Can you work these out from the model? Positions are in its coordinate system, mm. A direction names the side the tool comes from. Give positions to 0.01 mm unless a question says otherwise; leave off trailing zeros. Order: outer loops, then holes, each group sorted by start corner. A loop starts at its lowest first (then second) coordinate and runs counter-clockwise, first axis right, second up.
Item 1: I want a section at C-C, the plane x = 35. Write out the boundary of the cut face in (y, z), then the cut area to 3 significant figures.
Item 2: I want a section at B-B, the plane z = -20. Write out the boundary of the cut face in (x, y).
Item 3: If I drill on line 1 along X through (y, z) = (36.5, -55); line 2 along Z through (x, y) = (18.5, 33.5); line 3 along Y through (x, z) = (26, -10), over which ranges is the centre line in solid material (lowest first)?
Item 4: Which directions (+Z, -Z, +X, -X, +Y, -Y) give clear straight access to the entire face, cutting with the end or side of a thin tool? Please do faces 4 (the flat face through (25, 32, -30)), 5 (the flat face through (8, 5, -30)), 6 (the flat face through (15, 32, -30)), 7 (the flat face through (32, 5, -30)).
Item 5: I want a section at D-D, the plane y = 6. Write out the boundary of the cut face in (x, z).
Item 6: I'm going to push flat-ended pins straight in: pin 1 Ø5.5 at (y, z) = (35.3, -46.5) entering from +X (1 decimal); pin 2 Ø4 at (x, y) = (9, 23.5) entering from +Z; pin 3 Ø2 at (x, z) = (10, -25) entering from +Y; pin 4 Ø8 at (x, z) = (30.5, -20.5) entering from +Y. Where does each tip first touch, or does it pass through?
Item 7: I want a section at A-A, the plane z = -30. Write out the boundary of the cut face in (x, y), then the cut area to 3 significant figures.
Item 8: If we mould it in two halves opening along Y, with no side actions, what happens to faces 1 (the flat face through (20, 0, -30)), 2 (the cylindrical face through (17.028, 38.166, -12.599)), 3 (the flat face through (19, 32, -30))? For each: +Y half, -Y half, draft (parallel to the pull), parting line (faces both ways), or undercut.
```python
from build123d import *

# Parameters (mm, degrees)
ESQUISSE1_W             = 40
ESQUISSE1_H             = 60
BOSS_EXTRU_1_DEPTH      = 5
BOSS_EXTRU_3_DEPTH      = 60
BOSS_EXTRU_5_START      = -60
BOSS_EXTRU_5_DEPTH      = 60
ESQUISSE5_R             = 3
ENL_V_MAT_EXTRU_1_DEPTH = 76.959376992


with BuildPart() as part:
    # Esquisse1 → Boss.-Extru.1 (new body)
    with BuildSketch(Plane(origin=(0, 0, 0), x_dir=(1, 0, 0), z_dir=(0, 1, 0))):
        with Locations((20, 30)):
            Rectangle(ESQUISSE1_W, ESQUISSE1_H)
    extrude(amount=BOSS_EXTRU_1_DEPTH)

    # Esquisse3 → Boss.-Extru.3 (add)
    with BuildSketch(Plane.XY.offset(-60)):
        with BuildLine():
            Line((16, 5), (16, 15))
            ThreePointArc((16, 15), (20, 13.710800302), (24, 15))
            Line((24, 15), (24, 5))
            Line((24, 5), (16, 5))
        make_face()
    extrude(amount=BOSS_EXTRU_3_DEPTH)

    # Esquisse4 → Boss.-Extru.5 (add)
    with BuildSketch(Plane.XY.offset(BOSS_EXTRU_5_START)):
        with BuildLine():
            Line((15, 31.304286701), (15, 39.304286701))
            Line((15, 39.304286701), (19, 39.304286701))
            Line((19, 39.304286701), (19, 27.337414501))
            ThreePointArc((19, 27.337414501), (20, 13.710800302), (21, 27.337414501))
            Line((21, 27.337414501), (21, 39.304286701))
            Line((21, 39.304286701), (25, 39.304286701))
            Line((25, 39.304286701), (25, 31.304286701))
            ThreePointArc((25, 31.304286701), (20, 8.710800302), (15, 31.304286701))
        make_face()
    extrude(amount=BOSS_EXTRU_5_DEPTH)

    # Esquisse5 → Enlèv. mat.-Extru.1 (cut, through all)
    with BuildSketch(Plane(origin=(25, 0, 0), x_dir=(0, 0, -1), z_dir=(1, 0, 0))):
        with Locations(Location((13.5, 35.304286701, 0), (0, 0, 90))):
            Circle(ESQUISSE5_R)
        with Locations(Location((30, 35.304286701, 0), (0, 0, 90))):
            Circle(ESQUISSE5_R)
        with Locations(Location((46.5, 35.304286701, 0), (0, 0, 90))):
            Circle(ESQUISSE5_R)
    extrude(amount=-ENL_V_MAT_EXTRU_1_DEPTH, mode=Mode.SUBTRACT)


solid = part.part
```
Results list:
1. outline: (0, -60) - (5, -60) - (5, 0) - (0, 0) - close
1. area: 300 mm2
2. outline: (0, 0) - (40, 0) - (40, 5) - (24, 5) - (24, 9.41) arc R11.85 ccw to (25, 31.3) - (25, 39.3) - (21, 39.3) - (21, 27.34) arc R6.85 cw (long way) to (19, 27.34) - (19, 39.3) - (15, 39.3) - (15, 31.3) arc R11.85 ccw to (16, 9.41) - (16, 5) - (0, 5) - close
3. line 1: x = 15 to 19, 21 to 25
3. line 2: z = -60 to -48.9, -44.1 to -32.4, -27.6 to -15.9, -11.1 to 0
3. line 3: y = 0 to 5, 10.34 to 17.26, 23.87 to 30.78
4. face 4: +Z, -Z, +X, +Y
4. face 5: +Z, -Z, -X
4. face 6: +Z, -Z, -X, +Y
4. face 7: +Z, -Z, +X
5. outline: (16, -60) - (24, -60) - (24, 0) - (16, 0) - close
6. pin 1: passes through
6. pin 2: stops at z = 0
6. pin 3: stops at y = 28.27
6. pin 4: stops at y = 30.47
7. outline: (0, 0) - (40, 0) - (40, 5) - (24, 5) - (24, 9.41) arc R11.85 ccw to (25, 31.3) - (25, 32.3) - (21, 32.3) - (21, 27.34) arc R6.85 cw (long way) to (19, 27.34) - (19, 32.3) - (15, 32.3) - (15, 31.3) arc R11.85 ccw to (16, 9.41) - (16, 5) - (0, 5) - close; (15, 38.3) - (19, 38.3) - (19, 39.3) - (15, 39.3) - close; (21, 38.3) - (25, 38.3) - (25, 39.3) - (21, 39.3) - close
7. area: 526 mm2
8. face 1: -Y half
8. face 2: undercut
8. face 3: draft
